Design review of the part built by this model. Coordinates are the model's own, in mm. Face numbers are marked on the shaded views. Round coordinates to 2 decimals unless told otherwise and drop trailing zeros. Loops run counter-clockwise (first coordinate to the right, second up) from the corner with the lowest first, then second, coordinate; pieces in that order, holes last. Notation, with made-up numbers: (53, -18.75) - (68, -18.75) arc R11 cw to (68, 0.25) - close; hole circle Ø5 at (78.5, 64). An arc over 180 degrees is marked (long way). Answer as CSV lines item,"result". Start each with the question number.
(1) Wall thickness on L1, parallel to X at y = -0.8, z = -35.45 (3 decimals); L2, parallel to X at y = 0.4, z = -35.45; L3, parallel to X at y = -0.25, z = 21: over which ranges is each line inside the solid? List them lowest first.
(2) Consider section C-C (x = 5). Give the boundary of the cut face in (y, z), and give its area (3 significant figures).
(3) For P1, Ø5.5, axis at x = 3.5, z = -35, coming from the -Y side; P2, Ø1.5, axis at x = -7.5, z = 4.5, coming from the -Y side; P3, Ø7, axis at x = -17, z = -6, coming from the -Y side, all flat-tipped, find the tip position at first contact; note any pin that passes through.
(4) Consider section A-A (z = -35.45). Give the boundary of the cut face in (x, y) (3 decimals), and give its area (4 significant figures).
(5) Consider section B-B (x = -4.5). Give the boundary of the cut face in (y, z) (3 decimals).
(6) Consider section D-D (z = 10). Give the boundary of the cut face in (x, y), and give its area (3 significant figures).
(7) Mouldability with a two-part tool opening along Z and no side actions: class the marked faces 1, 2 and 3 as released by +Z, released by -Z, zero draft, split by the parting line, or undercut.
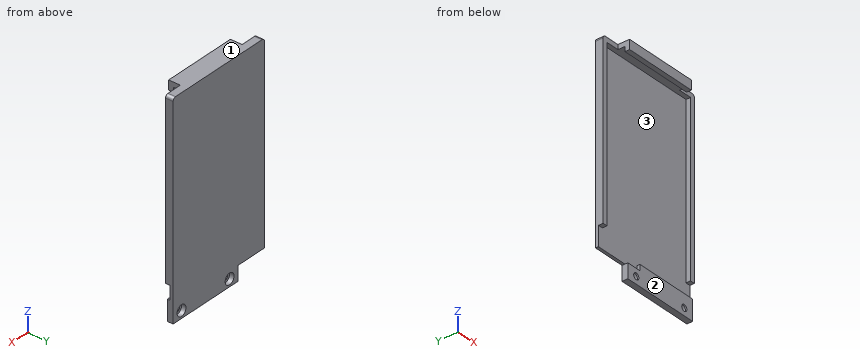
from build123d import *

# Parameters (mm, degrees)
SKETCH1_W                = 38
SKETCH1_H                = 65.9
BOSS_EXTRUDE1_DEPTH      = 1
BOSS_EXTRUDE2_DEPTH      = 1.58
SKETCH3_W                = 25.7
SKETCH3_H                = 1.6
BOSS_EXTRUDE3_DEPTH      = 4
SKETCH4_W                = 25.7
SKETCH4_H                = 1.6
BOSS_EXTRUDE4_DEPTH      = 1.6
FILLET1_R                = 1
SKETCH6_W                = 22
SKETCH6_H                = 7
BOSS_EXTRUDE5_DEPTH      = 1
BOSS_EXTRUDE5_DEPTH_BACK = 1
SKETCH9_W                = 5
SKETCH9_H                = 2
BOSS_EXTRUDE6_DEPTH      = 5
SKETCH7_R                = 1.075
CUT_EXTRUDE2_DEPTH       = 7.58
SKETCH8_R                = 1.85
CUT_EXTRUDE3_DEPTH       = 1.5


with BuildPart() as part:
    # Sketch1 → Boss-Extrude1 (new body)
    with BuildSketch(Plane(origin=(0, 0, 0), x_dir=(1, 0, 0), z_dir=(0, 1, 0))):
        Rectangle(SKETCH1_W, SKETCH1_H)
    extrude(amount=BOSS_EXTRUDE1_DEPTH)

    # Sketch2 → Boss-Extrude2 (add)
    with BuildSketch(Plane.XZ):
        Polygon((-19, 32.95), (-19, -26.25), (-17.4, -26.25), (-17.4, 31.35), (17.4, 31.35), (17.4, -26.25), (19, -26.25), (19, 32.95), align=None)
    extrude(amount=BOSS_EXTRUDE2_DEPTH)

    # Sketch3 → Boss-Extrude3 (add)
    with BuildSketch(Plane.XZ.offset(1.58)):
        with Locations((0, 32.15)):
            Rectangle(SKETCH3_W, SKETCH3_H)
    extrude(amount=BOSS_EXTRUDE3_DEPTH)

    # Sketch4 → Boss-Extrude4 (add)
    with BuildSketch(Plane(origin=(0, 0, 31.35), x_dir=(-1, 0, 0), z_dir=(0, 0, -1))):
        with Locations((0, -4.78)):
            Rectangle(SKETCH4_W, SKETCH4_H)
    extrude(amount=BOSS_EXTRUDE4_DEPTH)

    # Fillet1
    fillet1_edges = [part.edges().sort_by_distance(p)[0] for p in [
        (19, -0.29, 32.95),
        (-19, -0.29, 32.95),
    ]]
    fillet(fillet1_edges, radius=FILLET1_R)

    # Sketch6 → Boss-Extrude5 (add, two sides)
    with BuildSketch(Plane.XZ) as boss_extrude5_sk:
        with Locations((8, -34.45)):
            Rectangle(SKETCH6_W, SKETCH6_H)
    extrude(amount=BOSS_EXTRUDE5_DEPTH)
    extrude(boss_extrude5_sk.sketch, amount=-BOSS_EXTRUDE5_DEPTH_BACK)

    # Sketch9 → Boss-Extrude6 (add)
    with BuildSketch(Plane.ZY.offset(3)):
        with Locations((-35.45, 0)):
            Rectangle(SKETCH9_W, SKETCH9_H)
    extrude(amount=BOSS_EXTRUDE6_DEPTH)

    # Sketch7 → Cut-Extrude2 (cut, through all)
    with BuildSketch(Plane(origin=(0, 1, 0), x_dir=(1, 0, 0), z_dir=(0, 1, 0))):
        with Locations((-4.5, 35.45)):
            Circle(SKETCH7_R)
        with Locations((15.5, 35.45)):
            Circle(SKETCH7_R)
    extrude(amount=-CUT_EXTRUDE2_DEPTH, mode=Mode.SUBTRACT)

    # Sketch8 → Cut-Extrude3 (cut)
    with BuildSketch(Plane(origin=(0, 1, 0), x_dir=(1, 0, 0), z_dir=(0, 1, 0))):
        with Locations((-4.5, 35.45)):
            Circle(SKETCH8_R)
        with Locations((15.5, 35.45)):
            Circle(SKETCH8_R)
    extrude(amount=-CUT_EXTRUDE3_DEPTH, mode=Mode.SUBTRACT)


solid = part.part
Determined:
1,L1,"x = -8 to -5.575, -3.425 to 14.425, 16.575 to 19"
1,L2,"x = -8 to -6.35, -2.65 to 13.65, 17.35 to 19"
1,L3,"x = -19 to -17.4, 17.4 to 19"
2,outline,"(-5.58, 29.75) - (-3.98, 29.75) - (-3.98, 31.35) - (0, 31.35) - (0, -30.95) - (-1, -30.95) - (-1, -37.95) - (1, -37.95) - (1, 32.95) - (-5.58, 32.95) - close"
2,area,"89.4 mm^2"
3,P1,"stops at y = -1"
3,P2,"stops at y = 0"
3,P3,"stops at y = -1.58"
4,outline,"(-8, -1) - (-5.575, -1) - (-5.575, -0.5) - (-6.35, -0.5) - (-6.35, 1) - (-8, 1) - close; (-3.425, -1) - (14.425, -1) - (14.425, -0.5) - (13.65, -0.5) - (13.65, 1) - (-2.65, 1) - (-2.65, -0.5) - (-3.425, -0.5) - close; (16.575, -1) - (19, -1) - (19, 1) - (17.35, 1) - (17.35, -0.5) - (16.575, -0.5) - close"
4,area,"40.75 mm^2"
5,outline,"(-5.58, 29.75) - (-3.98, 29.75) - (-3.98, 31.35) - (0, 31.35) - (0, -32.95) - (-1, -32.95) - (-1, -34.375) - (-0.5, -34.375) - (-0.5, -33.6) - (1, -33.6) - (1, 32.95) - (-5.58, 32.95) - close; (-1, -37.95) - (1, -37.95) - (1, -37.3) - (-0.5, -37.3) - (-0.5, -36.525) - (-1, -36.525) - close"
6,outline,"(-19, -1.58) - (-17.4, -1.58) - (-17.4, 0) - (17.4, 0) - (17.4, -1.58) - (19, -1.58) - (19, 1) - (-19, 1) - close"
6,area,"43.1 mm^2"
7,face 1,"released by +Z"
7,face 2,"zero draft"
7,face 3,"undercut"
